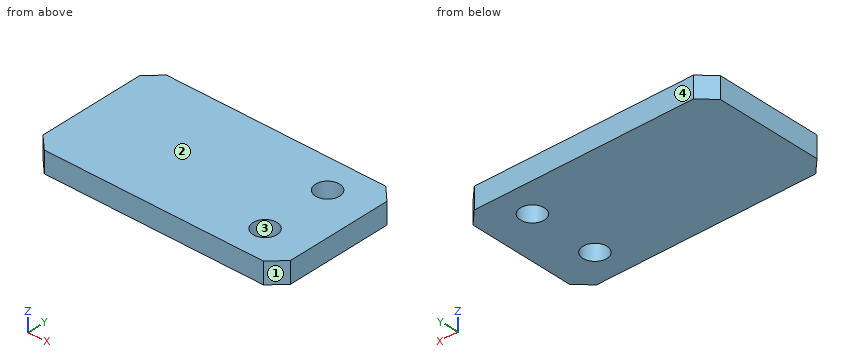
from build123d import *

# Parameters (mm, degrees)
SKETCH1_W                = 35
SKETCH1_H                = 19
BOSS_EXTRUDE1_DEPTH      = 3
CHAMFER1_SIZE            = 2
M3_CLEARANCE_HOLE1_D     = 3.4
M3_CLEARANCE_HOLE1_DEPTH = 3


with BuildPart() as part:
    # Sketch1 → Boss-Extrude1 (new body)
    with BuildSketch(Plane.XY):
        Rectangle(SKETCH1_W, SKETCH1_H)
    extrude(amount=BOSS_EXTRUDE1_DEPTH)

    # Chamfer1
    chamfer1_edges = [part.edges().sort_by_distance(p)[0] for p in [
        (17.5, -9.5, 1.5),
        (-17.5, -9.5, 1.5),
        (-17.5, 9.5, 1.5),
        (17.5, 9.5, 1.5),
    ]]
    chamfer(chamfer1_edges, length=CHAMFER1_SIZE)

    # M3 Clearance Hole1
    with Locations(Plane.XY.offset(3)):
        with Locations((11.5, 4.866311679), (11.5, -4.866311679)):
            Hole(M3_CLEARANCE_HOLE1_D / 2, depth=M3_CLEARANCE_HOLE1_DEPTH)


solid = part.part
Verification items for the finished model (mm, model axes). Face numbers are marked on the shaded views. Round coordinates to 2 decimals unless told otherwise and drop trailing zeros. Loops run counter-clockwise (first coordinate to the right, second up) from the corner with the lowest first, then second, coordinate; pieces in that order, holes last. Notation, with made-up numbers: (73.25, 37) - (120.25, 37) arc R19 ccw to (120.25, 54) - close; hole circle Ø4 at (63, 72.25). An arc over 180 degrees is marked (long way). Answer in a Markdown table with one row per item. Add a question column.
Q1. Section check A-A on x = 11.5. Enter the section's corners in (y, z), plus the area to 3 significant figures.
Q2. Section check C-C on y = 3.5. Enter the section's corners in (x, z).
Q3. Section check B-B on z = 2.6. Enter the section's corners in (x, y), plus the area to 3 significant figures.
Q4. Section check D-D on y = 8.25. Enter the section's corners in (x, z).
Q5. Release check for a two-part mould opening along Y. For the marked faces 1, 2, 3 and 4 record: pulls with the +Y half, pulls with the -Y half, needs draft (parallel to the pull), parting line crosses it, or undercut.
Q6. Gauge pin test, flat end, axial feed: pin 1 (3 mm diameter, centred on x = 11.5, y = 4.87, fed in from +Z). Record the tip position at first contact, or that the pin passes through.
Q7. Material ranges on line 1 (Y direction, x = 11.5, z = 2.35); line 2 (Y direction, x = 10, z = 1.8); line 3 (X direction, y = 5.25, z = 1.95), recorded low to high.
Found:
| question | item | result |
|---|---|---|
| 1 | outline | (-9.5, 0) - (-6.57, 0) - (-6.57, 3) - (-9.5, 3) - close; (-3.17, 0) - (3.17, 0) - (3.17, 3) - (-3.17, 3) - close; (6.57, 0) - (9.5, 0) - (9.5, 3) - (6.57, 3) - close |
| 1 | area | 36.6 mm² |
| 2 | outline | (-17.5, 0) - (10.49, 0) - (10.49, 3) - (-17.5, 3) - close; (12.51, 0) - (17.5, 0) - (17.5, 3) - (12.51, 3) - close |
| 3 | outline | (-17.5, -7.5) - (-15.5, -9.5) - (15.5, -9.5) - (17.5, -7.5) - (17.5, 7.5) - (15.5, 9.5) - (-15.5, 9.5) - (-17.5, 7.5) - close; hole circle Ø3.4 at (11.5, -4.87); hole circle Ø3.4 at (11.5, 4.87) |
| 3 | area | 639 mm² |
| 4 | outline | (-16.75, 0) - (16.75, 0) - (16.75, 3) - (-16.75, 3) - close |
| 5 | face 1 | pulls with the -Y half |
| 5 | face 2 | needs draft |
| 5 | face 3 | undercut |
| 5 | face 4 | pulls with the +Y half |
| 6 | pin 1 | passes through |
| 7 | line 1 | y = -9.5 to -6.57, -3.17 to 3.17, 6.57 to 9.5 |
| 7 | line 2 | y = -9.5 to -5.67, -4.07 to 4.07, 5.67 to 9.5 |
| 7 | line 3 | x = -17.5 to 9.84, 13.16 to 17.5 |
